For this review, take the finished solid that the model builds, in its own axes (mm). A direction names the side the tool comes from. Round coordinates to 2 decimals unless told otherwise and drop trailing zeros. Order: outer loops, then holes, each group sorted by start corner. A loop starts at its lowest first (then second) coordinate and runs counter-clockwise, first axis right, second up. Notation, with made-up numbers: (-9.5, 13) - (47.5, 13) arc R16 cw to (47.5, 34) - close; hole circle Ø2 at (-22, 13.25). An arc over 180 degrees is marked (long way). One line per item, written item: value.
```python
from build123d import *

# Parameters (mm, degrees)
F1_DEPTH = 15
F2_D     = 5.2
F3_D     = 10
F5_D     = 8.2
F7_D     = 11
F7_DEPTH = 5
F7_TIP   = 3.3047334047


with BuildPart() as f1:
    # F0 (on Top) → F1 (new body)
    with BuildSketch(Plane.XY):
        with BuildLine():
            Line((25, 13), (-25, 13))
            Line((-25, 13), (-25, -4))
            Line((-25, -4), (-18, -12))
            Line((-18, -12), (-30, -22))
            Line((-30, -22), (-30, -30))
            ThreePointArc((-30, -30), (-29.4142135624, -31.4142135624), (-28, -32))
            Line((-28, -32), (-15, -32))
            Line((-15, -32), (-15, -29))
            Line((-15, -29), (3, -29))
            Line((3, -29), (3, -12))
            Line((3, -12), (25, -12))
            Line((25, -12), (25, 13))
        make_face()
    extrude(amount=F1_DEPTH)

    # F2 (through all)
    with Locations(Plane(origin=(0, 0, 0), x_dir=(1, 0, 0), z_dir=(0, 0, -1))):
        with Locations((-15, 0), (15, 0)):
            Hole(F2_D / 2)

    # F3 (through all)
    with Locations(Plane(origin=(0, 0, 0), x_dir=(1, 0, 0), z_dir=(0, 0, -1))):
        with Locations((0, 0)):
            Hole(F3_D / 2)

    # F5 (through all)
    with Locations(Plane(origin=(-1.4754098361, 1.7704918033, 0), x_dir=(-0.7682212796, -0.6401843997, 0), z_dir=(-0.6401843997, 0.7682212796, 0))):
        with Locations((29.0101958287, 7.5)):
            Hole(F5_D / 2)

    # F7
    with Locations(Plane.YZ.offset(3)):
        with Locations((-22.5, 7.5376075692)):
            Hole(F7_D / 2, depth=F7_DEPTH)
            with Locations((0, 0, -(F7_DEPTH + F7_TIP / 2))):  # 118° drill point
                Cone(0, F7_D / 2, F7_TIP, mode=Mode.SUBTRACT)


solid = f1.part
```
Item 1: The part is to be moulded in two halves that separate along Z. For faces 6 (the conical face through (-4.73, -21.59, 7.82)), 7 (the flat face through (-22, -32, 7)), 8 (the flat face through (-3, -9, 0)), say which applies: +Z half, -Z half, draft (parallel to the pull), parting line (faces both ways), or undercut.
Returned:
face 6: undercut
face 7: draft
face 8: -Z half
Item 2: Take a section at C-C (x = 15). Write out the cut boundary in (y, z).
Returned:
outline: (-12, 0) - (-2.6, 0) - (-2.6, 15) - (-12, 15) - close; (2.6, 0) - (13, 0) - (13, 15) - (2.6, 15) - close
Item 3: Take a section at B-B (y = 0). Write out the cut boundary in (x, z), plus the area to 3 significant figures.
Returned:
outline: (-25, 0) - (-17.6, 0) - (-17.6, 15) - (-25, 15) - close; (-12.4, 0) - (-5, 0) - (-5, 15) - (-12.4, 15) - close; (5, 0) - (12.4, 0) - (12.4, 15) - (5, 15) - close; (17.6, 0) - (25, 0) - (25, 15) - (17.6, 15) - close
area: 444 mm^2
Item 4: Wall thickness on line 1 (Z direction, x = 1.1, y = -22.5); line 2 (X direction, y = 1, z = 8.75); line 3 (Y direction, x = 0, z = 4.5): over which ranges is each line inside the solid? List them lowest first.
Returned:
line 1: 0 to 2.04, 13.04 to 15
line 2: -25 to -17.4, -12.6 to -4.9, 4.9 to 12.6, 17.4 to 25
line 3: -29 to -27.09, -17.91 to -5, 5 to 13
Item 5: Machinability: for faces 1 (the cylindrical face through (-29.43, -31.4, 7.4)), 2 (the flat face through (-25, 5, 7)), 3 (the flat face through (-21.55, -7.94, 7.4)), 4 (the flat face through (-15, -31, 2)), 5 (the cylindrical face through (0.465, -25.457, 12.175)), which of the approach directions +Z, -Z, +X, -X, +Y, -Y give a long, thin tool a straight path to every point of the face, cutting with its end or side? Answer none if there is none.
Returned:
face 1: +Z, -Z, -X, -Y
face 2: +Z, -Z, -X, +Y
face 3: +Z, -Z, -X
face 4: +Z, -Z, +X, -Y
face 5: +X
Item 6: For P1, Ø4.5, axis at y = 5, z = 11, coming from the -X side; P2, Ø8, axis at x = 10, z = 8.5, coming from the -Y side; P3, Ø7.5, axis at x = -6, z = 6.5, coming from the -Y side, all flat-tipped, find the tip position at first contact; note any pin that passes through.
Returned:
P1: x = -25
P2: y = -12
P3: y = -29
Item 7: Take a section at A-A (x = 0). Write out the cut boundary in (y, z), plus the area to 3 significant figures.
Returned:
outline: (-29, 0) - (-5, 0) - (-5, 15) - (-29, 15) - close; (5, 0) - (13, 0) - (13, 15) - (5, 15) - close; hole circle Ø11 at (-22.5, 7.54)
area: 385 mm^2
